```python
from build123d import *

# Parameters (mm, degrees)
SKETCH1_W           = 110
SKETCH1_H           = 110
BOSS_EXTRUDE1_DEPTH = 5
SKETCH2_R           = 21.075
SKETCH2_R_2         = 18.025
BOSS_EXTRUDE2_DEPTH = 130
CHAMFER1_SIZE       = 2


with BuildPart() as part:
    # Sketch1 → Boss-Extrude1 (new body)
    with BuildSketch(Plane(origin=(0, 0, 0), x_dir=(1, 0, 0), z_dir=(0, 1, 0))):
        Rectangle(SKETCH1_W, SKETCH1_H)
    extrude(amount=BOSS_EXTRUDE1_DEPTH)

    # Sketch2 → Boss-Extrude2 (add)
    with BuildSketch(Plane(origin=(0, 5, 0), x_dir=(1, 0, 0), z_dir=(0, 1, 0))):
        with Locations(Location((0, 0, 0), (0, 0, 270))):
            Circle(SKETCH2_R)
        with Locations(Location((0, 0, 0), (0, 0, 270))):
            Circle(SKETCH2_R_2, mode=Mode.SUBTRACT)
    extrude(amount=BOSS_EXTRUDE2_DEPTH)

    # Chamfer1
    chamfer1_edges = [part.edges().sort_by_distance(p)[0] for p in [
        (0, 5, -21.075),
    ]]
    chamfer(chamfer1_edges, length=CHAMFER1_SIZE)


solid = part.part
```
Verification items for the finished model (mm, model axes). A direction names the side the tool comes from. Round coordinates to 2 decimals unless told otherwise and drop trailing zeros. Order: outer loops, then holes, each group sorted by start corner. A loop starts at its lowest first (then second) coordinate and runs counter-clockwise, first axis right, second up. Notation, with made-up numbers: (58.25, -12.75) -> (81.25, -12.75) arc R21 ccw to (81.25, 1.25) -> close; hole circle Ø1 at (5, 35.25). An arc over 180 degrees is marked (long way). Put each result on its own line as item: value. Start each with the question number.
(1) Section check B-B (z = 0). Enter the section's corners in (x, y) (3 decimals), then the cut area to 3 significant figures.
(2) Section check C-C (y = 101). Enter the section's corners in (x, z) (3 decimals), then the cut area to 3 significant figures.
(3) Material ranges on line 1 along X through (y, z) = (75.5, 0) (3 decimals); line 2 along Y through (x, z) = (-42.5, 16); line 3 along X through (y, z) = (98, -8), recorded low to high.
(4) Draft check along Z on faces 1 (the face through (55, 2, 1)), 2 (the face through (0, 5, 0)), 3 (the face through (-1, 2, 55)), 4 (the face through (-12.824, 70.104, -16.724)). Enter one of: +Z half, -Z half, draft (parallel to the pull), parting line (faces both ways), or undercut.
(5) Section check D-D (z = 27). Enter the section's corners in (x, y), then the cut area to 3 significant figures.
(6) Tool access check on faces 5 (the face through (-1, 2, -55)), 6 (the face through (-25, 5, -1)). Record the directions out of +Z, -Z, +X, -X, +Y, -Y that give a thin tool (end or side, any length) a straight path to the whole face; none if there is none.
(7) Section check A-A (x = 0). Enter the section's corners in (y, z) (3 decimals).
(8) Depth check by flat-ended pin: pin 1 Ø1 at (x, y) = (14, 102) entering from -Z; pin 2 Ø3 at (y, z) = (94.5, 24.5) entering from +X; pin 3 Ø4 at (y, z) = (81, 20.5) entering from +X; pin 4 Ø10 at (x, y) = (-4.5, 28.5) entering from +Z (3 decimals). Enter the tip coordinate at first touch or a pass-through.
Completed:
1. outline: (-55, 0) -> (55, 0) -> (55, 5) -> (23.075, 5) -> (21.075, 7) -> (21.075, 135) -> (18.025, 135) -> (18.025, 5) -> (-18.025, 5) -> (-18.025, 135) -> (-21.075, 135) -> (-21.075, 7) -> (-23.075, 5) -> (-55, 5) -> close
1. area: 1,350 mm2
2. outline: circle Ø42.15 at (0, 0); hole circle Ø36.05 at (0, 0)
2. area: 375 mm2
3. line 1: x = -21.075 to -18.025, 18.025 to 21.075
3. line 2: y = 0 to 5
3. line 3: x = -19.5 to -16.15, 16.15 to 19.5
4. face 1: draft
4. face 2: undercut
4. face 3: +Z half
4. face 4: parting line
5. outline: (-55, 0) -> (55, 0) -> (55, 5) -> (-55, 5) -> close
5. area: 550 mm2
6. face 5: -Z, +X, -X, +Y, -Y
6. face 6: +Y
7. outline: (0, -55) -> (5, -55) -> (5, -23.075) -> (7, -21.075) -> (135, -21.075) -> (135, -18.025) -> (5, -18.025) -> (5, 18.025) -> (135, 18.025) -> (135, 21.075) -> (7, 21.075) -> (5, 23.075) -> (5, 55) -> (0, 55) -> close
8. pin 1: stops at z = -16.18
8. pin 2: passes through
8. pin 3: stops at x = 10.09
8. pin 4: stops at z = 21.075
